Read the model definition and answer for the solid it produces. Units are mm, in the model's axes. Face numbers are marked on the shaded views. Round coordinates to 2 decimals unless told otherwise and drop trailing zeros. Use a Markdown table: item, result. Add a question column.
1. Given pin 1 (4 mm diameter, centred on x = 44.45, z = 0, fed in from +Y); pin 2 (2 mm diameter, centred on x = 5, z = -2, fed in from -Y), each flat-ended and moving along its own axis, determine where each tip first touches the part or whether it passes through.
2. Consider L1, parallel to X at y = 4, z = 0; L2, parallel to X at y = 3, z = -3; L3, parallel to X at y = 5.25, z = -2. Determine where each line is inside the solid, lowest interval first. Write a range as [from, to].
3. The mould has two halves that part along Z. Classify the marked faces 1, 2 and 3: +Z half, -Z half, draft (parallel to the pull), parting line (faces both ways), or undercut.
4. Section A-A, the plane y = 1.25 is taken. Give the number of separate pieces and of enclosed holes in the cut face, then the cut area to 3 significant figures.
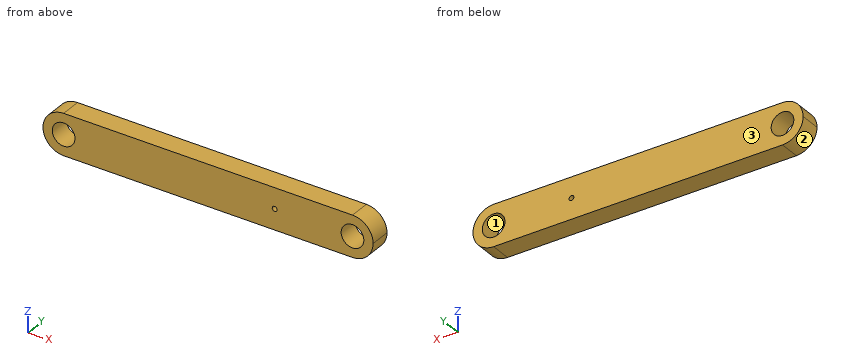
```python
from build123d import *

# Parameters (mm, degrees)
SKETCH1_R           = 3.4925
BOSS_EXTRUDE1_DEPTH = 6.35
FILLET1_R           = 6.35
SKETCH3_R           = 0.75
CUT_EXTRUDE1_DEPTH  = 52.587643869


with BuildPart() as part:
    # Sketch1 → Boss-Extrude1 (new body)
    with BuildSketch(Plane(origin=(0, 0, 0), x_dir=(1, 0, 0), z_dir=(0, 1, 0))):
        Polygon((-50.8, 6.35), (-50.8, -6.35), (-6.35, -6.35), (6.35, -6.35), (50.8, -6.35), (50.8, 6.35), (6.35, 6.35), (-6.35, 6.35), align=None)
        with Locations(Location((-44.45, 0, 0), (0, 0, 270))):
            Circle(SKETCH1_R, mode=Mode.SUBTRACT)
        with Locations(Location((44.45, 0, 0), (0, 0, 270))):
            Circle(SKETCH1_R, mode=Mode.SUBTRACT)
    extrude(amount=BOSS_EXTRUDE1_DEPTH)

    # Fillet1
    fillet1_edges = [part.edges().sort_by_distance(p)[0] for p in [
        (50.8, 3.175, -6.35),
        (-50.8, 3.175, -6.35),
        (-50.8, 3.175, 6.35),
        (50.8, 3.175, 6.35),
    ]]
    fillet(fillet1_edges, radius=FILLET1_R - 0.0001)  # a hair under: the kernel refuses the full size

    # Sketch3 → Cut-Extrude1 (cut, through all)
    with BuildSketch(Plane(origin=(0, 6.35, 0), x_dir=(1, 0, 0), z_dir=(0, 1, 0))):
        with Locations(Location((20.5, 0, 0), (0, 0, 270))):
            Circle(SKETCH3_R)
    extrude(amount=-CUT_EXTRUDE1_DEPTH, mode=Mode.SUBTRACT)


solid = part.part
```
Verdict:
| question | item | result |
|---|---|---|
| 1 | pin 1 | passes through |
| 1 | pin 2 | stops at y = 0 |
| 2 | L1 | x = [-50.8, -47.94], [-40.96, 19.75], [21.25, 40.96], [47.94, 50.8] |
| 2 | L2 | x = [-50.05, -46.24], [-42.66, 42.66], [46.24, 50.05] |
| 2 | L3 | x = [-50.48, -47.31], [-41.59, 41.59], [47.31, 50.48] |
| 3 | face 1 | undercut |
| 3 | face 2 | -Z half |
| 3 | face 3 | draft |
| 4 | separate pieces | 1 |
| 4 | enclosed holes | 3 |
| 4 | area | 1,180 mm2 |
